Part model, mm, in its own coordinate system. A direction names the side the tool comes from. Round coordinates to 2 decimals unless told otherwise and drop trailing zeros. Write each loop counter-clockwise with the first axis right and the second up, starting at its lowest first coordinate (ties: lowest second). Pieces come first, ordered by that corner, then holes.
```python
from build123d import *

# Parameters (mm, degrees)
F0_W      = 127
F0_H      = 127
F1_DEPTH  = 12.7
F2_W      = 114.3
F2_H      = 114.3
F2_W_2    = 63.5
F2_H_2    = 63.5
F3_DEPTH  = 6.35
F3_FACE_W = 63.5
F3_FACE_H = 63.5
F4_DEPTH  = 12.7


with BuildPart() as f1:
    # F0 (on Top) → F1 (new body)
    with BuildSketch(Plane.XY):
        Rectangle(F0_W, F0_H)
    extrude(amount=F1_DEPTH)

    # F2 (on face) → F3 (cut)
    with BuildSketch(Plane.XY.offset(12.7)):
        Rectangle(F2_W, F2_H)
        Rectangle(F2_W_2, F2_H_2, mode=Mode.SUBTRACT)
    extrude(amount=-F3_DEPTH, mode=Mode.SUBTRACT)

    # F3_face (on face) → F4 (join)
    with BuildSketch(Plane.XY.offset(12.7)):
        Rectangle(F3_FACE_W, F3_FACE_H)
    extrude(amount=F4_DEPTH)


solid = f1.part
```
Q1. Cut at A-A on x = 19. Write the cut outline in (y, z).
Values follow:
outline: (-63.5, 0) - (63.5, 0) - (63.5, 12.7) - (57.15, 12.7) - (57.15, 6.35) - (31.75, 6.35) - (31.75, 25.4) - (-31.75, 25.4) - (-31.75, 6.35) - (-57.15, 6.35) - (-57.15, 12.7) - (-63.5, 12.7) - close
Q2. Cut at C-C on z = 15.25. Write the cut outline in (x, y).
Values follow:
outline: (-31.75, -31.75) - (31.75, -31.75) - (31.75, 31.75) - (-31.75, 31.75) - close
Q3. Which spindle directions (+Z, -Z, +X, -X, +Y, -Y) get a long thin tool onto all of the face, cutting with end or side? Do faces 4 (the flat face through (-1, 1, 0)), 5 (the flat face through (-1, -57.15, 10)). Say none if no direction does.
Values follow:
face 4: -Z, +X, -X, +Y, -Y
face 5: +Z
Q4. Wall check: L1, parallel to X at y = -23.5, z = 12; L2, parallel to Y at x = -12.5, z = 22. Give the ranges that are in metal, low to high.
Values follow:
L1: x = -63.5 to -57.15, -31.75 to 31.75, 57.15 to 63.5
L2: y = -31.75 to 31.75
Q5. Mould opens along Y. For faces 1 (the flat face through (31.75, 0, 16)), 2 (the flat face through (-63.5, -1, 6)), 3 (the flat face through (-1, -63.5, 6)) say: +Y half, -Y half, draft (parallel to the pull), parting line (faces both ways), or undercut.
Values follow:
face 1: undercut
face 2: draft
face 3: -Y half
Q6. Cut at B-B on y = 40.5. Write the cut outline in (x, z).
Values follow:
outline: (-63.5, 0) - (63.5, 0) - (63.5, 12.7) - (57.15, 12.7) - (57.15, 6.35) - (-57.15, 6.35) - (-57.15, 12.7) - (-63.5, 12.7) - close
Q7. Drop a flat-ended pin along its axis: pin 1 (1 mm diameter, centred on x = -26, z = 17, fed in from +Y). Give the stop position or say it passes through.
Values follow:
pin 1: stops at y = 31.75
